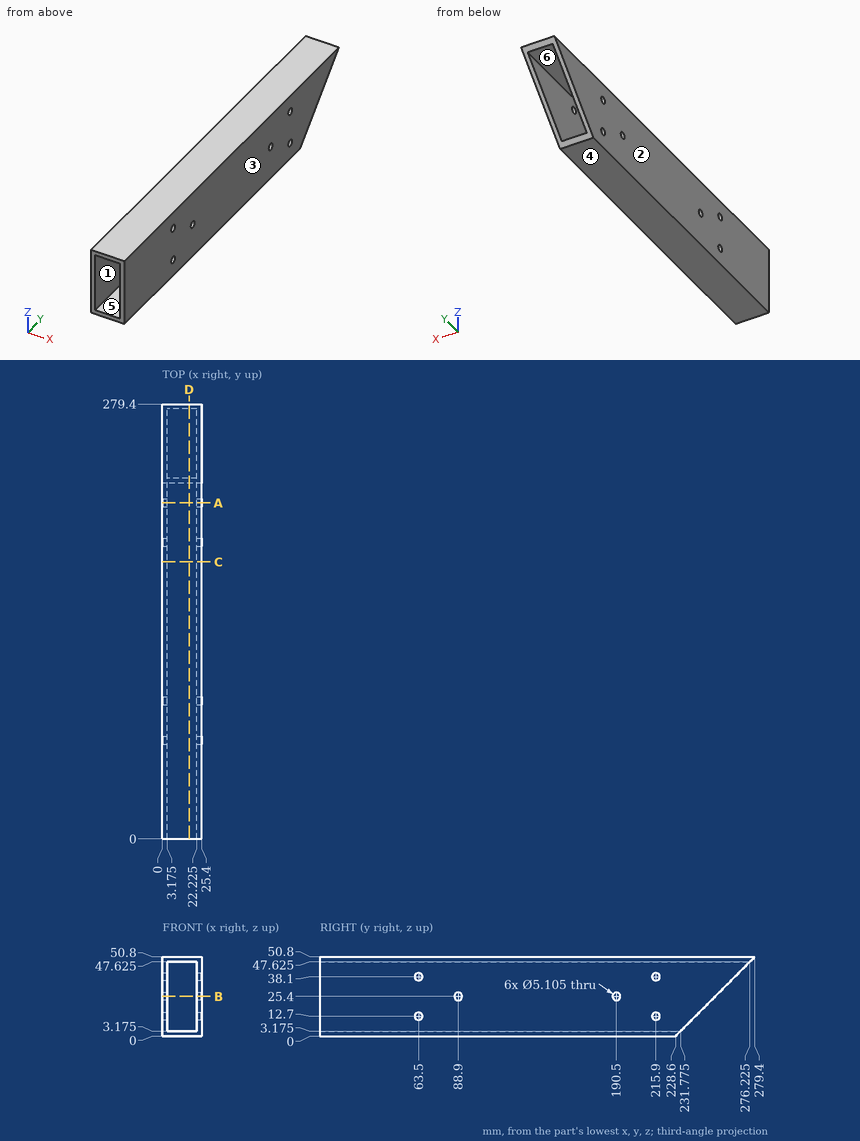
The drawing under review shows one solid part. Ordinate dimensions are in mm from its lowest x, y, z. A direction names the side the tool comes from. Round coordinates to 2 decimals unless told otherwise and drop trailing zeros. Write each loop counter-clockwise with the first axis right and the second up, starting at its lowest first coordinate (ties: lowest second). Pieces come first, ordered by that corner, then holes. Notation, with made-up numbers: M 51.5,62.25 L 92.5,62.25 A30 ccw 92.5,86.25 Z; hole C 72,62 d3. An arc over 180 degrees is marked long. One line per item, written item: value. Start each with the question number.
(1) We need section D-D (x = 17.25). Give the boundary of the cut face in (y, z) (1 decimal), and give its area (3 significant figures).
(2) The part is to be moulded in two halves that separate along Z. For the marked faces 3, 4, 5 and 6, say which applies: released by +Z, released by -Z, zero draft, split by the parting line, or undercut.
(3) We need section C-C (y = 178). Give the boundary of the cut face in (x, z) (1 decimal).
(4) We need section B-B (z = 25.4). Give the boundary of the cut face in (x, y) (1 decimal).
(5) We need section A-A (y = 215.9). Give the boundary of the cut face in (x, z) (1 decimal).
(6) Machinability: for the marked faces 1 and 2, which of the approach directions +Z, -Z, +X, -X, +Y, -Y give a long, thin tool a straight path to every point of the face, cutting with its end or side? Answer none if there is none.
(7) Wall thickness on line 1 (Z direction, x = 24.55, y = 215.9); line 2 (X direction, y = 33, z = 23.5) (1 decimal); line 3 (Z direction, x = 10.75, y = 202.5) (1 decimal): over which ranges is each line inside the solid? List them lowest first.
Result:
1. outline: M 0,0 L 228.6,0 L 231.8,3.2 L 0,3.2 Z; M 0,47.6 L 276.2,47.6 L 279.4,50.8 L 0,50.8 Z
1. area: 1,610 mm²
2. face 3: zero draft
2. face 4: released by -Z
2. face 5: undercut
2. face 6: undercut
3. outline: M 0,0 L 25.4,0 L 25.4,50.8 L 0,50.8 Z; hole M 3.2,3.2 L 22.2,3.2 L 22.2,47.6 L 3.2,47.6 Z
4. outline: M 0,0 L 3.2,0 L 3.2,86.3 L 0,86.3 Z; M 0,91.5 L 3.2,91.5 L 3.2,187.9 L 0,187.9 Z; M 0,193.1 L 3.2,193.1 L 3.2,254 L 0,254 Z; M 22.2,0 L 25.4,0 L 25.4,86.3 L 22.2,86.3 Z; M 22.2,91.5 L 25.4,91.5 L 25.4,187.9 L 22.2,187.9 Z; M 22.2,193.1 L 25.4,193.1 L 25.4,254 L 22.2,254 Z
5. outline: M 0,0 L 25.4,0 L 25.4,10.1 L 22.2,10.1 L 22.2,3.2 L 3.2,3.2 L 3.2,10.1 L 0,10.1 Z; M 0,15.3 L 3.2,15.3 L 3.2,35.5 L 0,35.5 Z; M 0,40.7 L 3.2,40.7 L 3.2,47.6 L 22.2,47.6 L 22.2,40.7 L 25.4,40.7 L 25.4,50.8 L 0,50.8 Z; M 22.2,15.3 L 25.4,15.3 L 25.4,35.5 L 22.2,35.5 Z
6. face 1: +Y, -Y
6. face 2: +Z, -Z, -X, +Y, -Y
7. line 1: 0 to 10.15, 15.25 to 35.55, 40.65 to 50.8
7. line 2: 0 to 3.2, 22.2 to 25.4
7. line 3: 0 to 3.2, 47.6 to 50.8
